Geometry check sheet. Reference: the model listing, model coordinates, mm. A direction names the side the tool comes from. Give positions to 0.01 mm unless a question says otherwise; leave off trailing zeros. Write each loop counter-clockwise with the first axis right and the second up, starting at its lowest first coordinate (ties: lowest second). Pieces come first, ordered by that corner, then holes. Notation, with made-up numbers: (65, -34) -> (98, -34) arc R14 ccw to (98, -14) -> close; hole circle Ø6 at (53.5, 87.25). An arc over 180 degrees is marked (long way). Write item = value, one per line. Start each with the question number.
1. Cross-section at C-C, the plane z = -2. Record the cut outline in (x, y).
2. Cross-section at B-B, the plane x = -55. Record the cut outline in (y, z), plus the area to 3 significant figures.
3. Cross-section at A-A, the plane y = -14.5. Record the cut outline in (x, z).
4. Set-up check for faces 4 (the flat face through (-55, -29, 0)), 5 (the flat face through (-5, 0, 2)), 6 (the flat face through (-60, -26, 1)): record each of +Z, -Z, +X, -X, +Y, -Y from which the full face is reachable in a straight line by a thin tool's end or side.
5. Mould release check, pull along Z, two halves, no side actions. Record for faces 1 (the flat face through (55, -29, 3)), 2 (the flat face through (0, 0, 0)), 3 (the flat face through (-1, 1.5, 4)): pulls with the +Z half, pulls with the -Z half, needs draft (parallel to the pull), parting line crosses it, or undercut.
6. Depth check by flat-ended pin: P1, Ø3.5, axis at x = 32.5, z = 1, coming from the -Y side; P2, Ø0.9, axis at y = -34.5, z = 2, coming from the +X side; P3, Ø3.5, axis at y = -30, z = 1.5, coming from the -X side. Enter the tip coordinate at first touch or a pass-through.
7. Thickness scan on line 1 along Y through (x, z) = (55, 2.1); line 2 along X through (y, z) = (-44, 1.5); line 3 along Y through (x, z) = (4, 4.5). Record the ranges inside material, lowest first.
```python
from build123d import *

# Parameters (mm, degrees)
SKETCH1_R           = 2.5
BOSS_EXTRUDE1_DEPTH = 3
SKETCH2_W           = 130
SKETCH2_H           = 12
BOSS_EXTRUDE2_DEPTH = 3
SKETCH3_W           = 10
SKETCH3_H           = 3
CUT_EXTRUDE1_DEPTH  = 3


with BuildPart() as part:
    # Sketch1 → Boss-Extrude1 (new body)
    with BuildSketch(Plane.XY):
        with BuildLine():
            Line((-50, -51.5), (-50, -1.5))
            Line((-50, -1.5), (50, -1.5))
            Line((50, -1.5), (50, -51.5))
            ThreePointArc((50, -51.5), (55, -56.5), (60, -51.5))
            Line((60, -51.5), (60, -1.5))
            Line((60, -1.5), (65, -1.5))
            Line((65, -1.5), (65, 1.5))
            Line((65, 1.5), (-65, 1.5))
            Line((-65, 1.5), (-65, -1.5))
            Line((-65, -1.5), (-60, -1.5))
            Line((-60, -1.5), (-60, -51.5))
            ThreePointArc((-60, -51.5), (-55, -56.5), (-50, -51.5))
        make_face()
        with Locations((-55, -51.5)):
            Circle(SKETCH1_R, mode=Mode.SUBTRACT)
        with Locations((55, -51.5)):
            Circle(SKETCH1_R, mode=Mode.SUBTRACT)
    extrude(amount=BOSS_EXTRUDE1_DEPTH)

    # Sketch2 → Boss-Extrude2 (add)
    with BuildSketch(Plane(origin=(0, 1.5, 0), x_dir=(1, 0, 0), z_dir=(0, 1, 0))):
        with Locations((0, -1.5)):
            Rectangle(SKETCH2_W, SKETCH2_H)
    extrude(amount=-BOSS_EXTRUDE2_DEPTH)

    # Sketch3 → Cut-Extrude1 (cut)
    with BuildSketch(Plane(origin=(0, 1.5, 0), x_dir=(1, 0, 0), z_dir=(0, 1, 0))):
        with Locations((0, -1.5)):
            Rectangle(SKETCH3_W, SKETCH3_H)
    extrude(amount=-CUT_EXTRUDE1_DEPTH, mode=Mode.SUBTRACT)


solid = part.part
```
Answers:
q1.outline = (-65, -1.5) -> (65, -1.5) -> (65, 1.5) -> (-65, 1.5) -> close
q2.outline = (-56.5, 0) -> (-54, 0) -> (-54, 3) -> (-56.5, 3) -> close; (-49, 0) -> (-1.5, 0) -> (-1.5, -4.5) -> (1.5, -4.5) -> (1.5, 7.5) -> (-1.5, 7.5) -> (-1.5, 3) -> (-49, 3) -> close
q2.area = 186 mm^2
q3.outline = (-60, 0) -> (-50, 0) -> (-50, 3) -> (-60, 3) -> close; (50, 0) -> (60, 0) -> (60, 3) -> (50, 3) -> close
q4.face_4 = -Z, +X, -X, -Y
q4.face_5 = +Y, -Y
q4.face_6 = +Z, -Z, -X, -Y
q5.face_1 = pulls with the +Z half
q5.face_2 = undercut
q5.face_3 = needs draft
q6.P1 = -1.5
q6.P2 = 60
q6.P3 = -60
q7.line_1 = -56.5 to -54, -49 to 1.5
q7.line_2 = -60 to -50, 50 to 60
q7.line_3 = -1.5 to 1.5
